from build123d import *

# Parameters (mm, degrees)
SKETCH1_R           = 16.8671875
BOSS_EXTRUDE1_DEPTH = 228.6
SKETCH2_W           = 7.9375
SKETCH2_H           = 3.175
FILLET1_R           = 3.175
CUT_EXTRUDE1_DEPTH  = 458.821847482


with BuildPart() as part:
    # Sketch1 → Boss-Extrude1 (new, symmetric)
    with BuildSketch(Plane.XY):
        Circle(SKETCH1_R)
    extrude(amount=BOSS_EXTRUDE1_DEPTH, both=True)

    # Sketch2 → Cut-Revolve1 (revolve, cut)
    with BuildSketch(Plane(origin=(0, 0, 0), x_dir=(1, 0, 0), z_dir=(0, 1, 0))):
        with Locations((12.8984375, -227.0125)):
            Rectangle(SKETCH2_W, SKETCH2_H)
        with Locations((12.8984375, 227.0125)):
            Rectangle(SKETCH2_W, SKETCH2_H)
    revolve(axis=Axis((0, 0, 0), (0, 0, -1)), mode=Mode.SUBTRACT)

    # Fillet1
    fillet1_edges = [part.edges().sort_by_distance(p)[0] for p in [
        (-16.8671875, 0, -225.425),
        (-16.8671875, 0, 225.425),
    ]]
    fillet(fillet1_edges, radius=FILLET1_R)

    # Sketch3 → Cut-Extrude1 (cut, through all)
    with BuildSketch(Plane.XY.offset(228.6)):
        Polygon((7.332348419, 0), (3.666174209, 6.35), (-3.666174209, 6.35), (-7.332348419, 0), (-3.666174209, -6.35), (3.666174209, -6.35), align=None)
    extrude(amount=-CUT_EXTRUDE1_DEPTH, mode=Mode.SUBTRACT)


solid = part.part
For this review, take the finished solid that the model builds, in its own axes (mm). A direction names the side the tool comes from. Round coordinates to 2 decimals unless told otherwise and drop trailing zeros. Write each loop counter-clockwise with the first axis right and the second up, starting at its lowest first coordinate (ties: lowest second). Pieces come first, ordered by that corner, then holes. Notation, with made-up numbers: M 73,81.25 L 123,81.25 A23 cw 123,106.25 Z; hole C 56,60.25 d4. An arc over 180 degrees is marked long. Write item = value, one per line. Start each with the question number.
(1) For line 1 along Z through (x, y) = (9.5, 9) (3 decimals); line 2 along X through (y, z) = (2.5, 87); line 3 along Y through (x, z) = (-3.5, -66.5), list the stretches that pass through material, from the lowest coordinate up.
(2) Clearance check with flat-ended pins moving along their axes: pin 1 Ø4 at (x, z) = (12, -43) entering from -Y; pin 2 Ø3 at (y, z) = (-12, 25.5) entering from -X; pin 3 Ø2 at (y, z) = (-7.5, 27.5) entering from -X; pin 4 Ø8 at (x, z) = (-0.5, 21) entering from +Y. State where each tip first meets the part, or that it passes through.
(3) For faces 1 (the face through (-8.92, -0.39, -227.03)), 2 (the face through (6, 3, 228.6)), 3 (the face through (-3, 9, 225.425)), list the 3-axis set-ups (+Z, -Z, +X, -X, +Y, -Y) from which the entire face can be reached by the end or side of a thin tool; tool diameter is ignored.
(4) We need section A-A (z = -129.5). Give the boundary of the cut face in (x, y).
(5) The part is to be moulded in two halves that separate along Y. For faces 4 (the face through (0, 6.35, 3)), 5 (the face through (6, 3, -228.6)), 6 (the face through (0, -6.35, 3)), 7 (the face through (-3.656, -16.466, 3.112)), say which applies: +Y half, -Y half, draft (parallel to the pull), parting line (faces both ways), or undercut.
Results found:
q1.line_1 = -225.425 to 225.425
q1.line_2 = -16.68 to -5.89, 5.89 to 16.68
q1.line_3 = -16.5 to -6.35, 6.35 to 16.5
q2.pin_1 = -13.58
q2.pin_2 = -13.2
q2.pin_3 = -15.56
q2.pin_4 = 16.87
q3.face_1 = -Z
q3.face_2 = +Z, +X, -X, +Y, -Y
q3.face_3 = +Z
q4.outline = C 0,0 d33.73; hole M -7.33,0 L -3.67,-6.35 L 3.67,-6.35 L 7.33,0 L 3.67,6.35 L -3.67,6.35 Z
q5.face_4 = undercut
q5.face_5 = draft
q5.face_6 = undercut
q5.face_7 = parting line
